The listing builds one solid part. Answer for the finished solid, in the listing's coordinates (mm). Face numbers are marked on the shaded views. A direction names the side the tool comes from. Give positions to 0.01 mm unless a question says otherwise; leave off trailing zeros. Order: outer loops, then holes, each group sorted by start corner. A loop starts at its lowest first (then second) coordinate and runs counter-clockwise, first axis right, second up. Notation, with made-up numbers: (60, 21.25) - (78, 21.25) arc R12 cw to (78, 33.25) - close; hole circle Ø1 at (66.5, -27). An arc over 180 degrees is marked (long way). Answer in a Markdown table with one row per item.
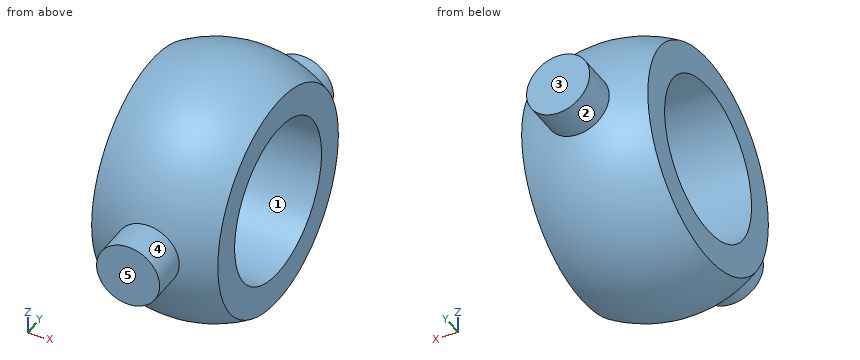
from build123d import *

# Parameters (mm, degrees)
F0_W = 80
F0_H = 30
F5_R = 20


with BuildPart() as f1:
    # F0 (on Front) → F1 (revolve)
    with BuildSketch(Plane.XZ):
        with Locations((0, 65)):
            Rectangle(F0_W, F0_H)
    revolve(axis=Axis((-190.0887642899, 0, 0), (-1, 0, 0)))

    # F2 (on Top) → F3 (revolve, cut)
    with BuildSketch(Plane.XY):
        with BuildLine():
            ThreePointArc((0, -80), (-80, 0), (0, 80))
            Line((0, 80), (0, 110))
            Line((0, 110), (-110, 110))
            Line((-110, 110), (-110, -110))
            Line((-110, -110), (0, -110))
            Line((0, -110), (0, -80))
        make_face()
    revolve(axis=Axis((0, 23.6749413657, 0), (0, 1, 0)), mode=Mode.SUBTRACT)

    # F5 (on offset) → F6 (join, up to the next surface of F1)
    with BuildSketch(Plane.XZ.offset(100)):
        Circle(F5_R)
    extrude(until=Until.NEXT, dir=(0, 1, 0))

    # F7: F1 across plane


with BuildPart() as f1_1:
    add(f1.part)
    add(f1.part.mirror(Plane.XZ))


solid = f1_1.part
Item 1: Find section A-A on y = 0. Write down the section's boundary in (x, z), then the cut area to 3 significant figures.
Answer block:
| item | result |
|---|---|
| outline | (-40, -69.28) arc R80 ccw to (40, -69.28) - (40, -50) - (-40, -50) - close; (-40, 50) - (40, 50) - (40, 69.28) arc R80 ccw to (-40, 69.28) - close |
| area | 4,240 mm² |
Item 2: Consider line 1 (Y direction, x = 10, z = 0); line 2 (Z direction, x = -21.5, y = 6); line 3 (Y direction, x = -9.5, z = -22). Determine where each line is inside the solid, lowest interval first.
Answer block:
| item | result |
|---|---|
| line 1 | -100 to -50, 50 to 100 |
| line 2 | -76.82 to -49.64, 49.64 to 76.82 |
| line 3 | -76.33 to -44.9, 44.9 to 76.33 |
Item 3: Find section D-D on y = 29. Write down the section's boundary in (x, z), then the cut area to 3 significant figures.
Answer block:
| item | result |
|---|---|
| outline | (-40, -62.92) arc R74.56 ccw to (40, -62.92) - (40, -40.73) - (-40, -40.73) - close; (-40, 40.73) - (40, 40.73) - (40, 62.92) arc R74.56 ccw to (-40, 62.92) - close |
| area | 4,810 mm² |
Item 4: Which of the six approach directions +Z, -Z, +X, -X, +Y, -Y give full straight-line access (tool end or side, diameter ignored) to the marked faces 4 and 5?
Answer block:
| item | result |
|---|---|
| face 4 | -Y |
| face 5 | +Z, -Z, +X, -X, -Y |
Item 5: Find section B-B on x = 0. Write down the section's boundary in (y, z), then the cut area to 3 significant figures.
Answer block:
| item | result |
|---|---|
| outline | (-100, -20) - (-77.46, -20) arc R80 ccw to (77.46, -20) - (100, -20) - (100, 20) - (77.46, 20) arc R80 ccw to (-77.46, 20) - (-100, 20) - close; hole circle Ø100 at (0, 0) |
| area | 13,900 mm² |
Item 6: Each of these flat-tipped pins is pushed along its axis until it touches: P1, Ø5, axis at x = 5, y = -46, coming from the -Z side; P2, Ø8, axis at x = 3, y = 75.5, coming from the -Z side; P3, Ø12, axis at x = -17, y = -17, coming from the -Z side. Where does it stop, or does it pass through?
Answer block:
| item | result |
|---|---|
| P1 | z = -66.96 |
| P2 | z = -35.77 |
| P3 | z = -77.94 |
Item 7: Find section C-C on z = 0. Write down the section's boundary in (x, y).
Answer block:
| item | result |
|---|---|
| outline | (-40, -69.28) arc R80 ccw to (-20, -77.46) - (-20, -100) - (20, -100) - (20, -77.46) arc R80 ccw to (40, -69.28) - (40, -50) - (-40, -50) - close; (-40, 50) - (40, 50) - (40, 69.28) arc R80 ccw to (20, 77.46) - (20, 100) - (-20, 100) - (-20, 77.46) arc R80 ccw to (-40, 69.28) - close |
Item 8: Determine the mould class of the marked faces 1, 2 and 3 for opening direction Y: pulls with the +Y half, pulls with the -Y half, needs draft (parallel to the pull), parting line crosses it, or undercut.
Answer block:
| item | result |
|---|---|
| face 1 | undercut |
| face 2 | needs draft |
| face 3 | pulls with the +Y half |
